Check sheet for the modelled part. Datum: model origin and axes. Units: mm. A direction names the side the tool comes from. Round coordinates to 2 decimals unless told otherwise and drop trailing zeros. Order: outer loops, then holes, each group sorted by start corner. A loop starts at its lowest first (then second) coordinate and runs counter-clockwise, first axis right, second up.
```python
from build123d import *

# Parameters (mm, degrees)
F0_W      = 50.8
F0_H      = 457.2
F1_DEPTH  = 25.4
F2_W      = 25.4
F2_H      = 50.8
F3_DEPTH  = 25.4
F4_W      = 25.4
F4_H      = 50.8
F5_DEPTH  = 431.8
F6_W      = 25.4
F6_H      = 50.8
F7_DEPTH  = 50.8
F8_W      = 50.8
F8_H      = 25.4
F9_DEPTH  = 406.4
F10_W     = 25.4
F10_H     = 50.8
F11_DEPTH = 25.4
F12_W     = 25.4
F12_H     = 50.8
F13_DEPTH = 431.8
F14_W     = 50.8
F14_H     = 50.8
F15_DEPTH = 25.4
F16_W     = 25.4
F16_H     = 50.8
F17_DEPTH = 381
F18_W     = 76.2
F18_H     = 50.8
F19_DEPTH = 25.4
F20_W     = 50.8
F20_H     = 25.4
F21_DEPTH = 406.4
F22_W     = 25.4
F22_H     = 50.8
F23_DEPTH = 406.4
F24_W     = 25.4
F24_H     = 50.8
F25_DEPTH = 431.8
F26_W     = 25.4
F26_H     = 50.8
F27_DEPTH = 406.4
F28_W     = 25.4
F28_H     = 50.8
F29_DEPTH = 25.4
F30_W     = 25.4
F30_H     = 50.8
F31_DEPTH = 431.8
F32_W     = 25.4
F32_H     = 50.8
F33_DEPTH = 431.8
F34_W     = 50.8
F34_H     = 50.8
F35_DEPTH = 25.4
F36_W     = 50.8
F36_H     = 25.4
F37_DEPTH = 406.4


with BuildPart() as f1:
    # F0 (on Front) → F1 (new body)
    with BuildSketch(Plane.XZ):
        with Locations((25.4, 228.6)):
            Rectangle(F0_W, F0_H)
    extrude(amount=F1_DEPTH)

    # F2 (on face) → F3 (join)
    with BuildSketch(Plane.YZ.offset(50.8)):
        with Locations((-12.7, 431.8)):
            Rectangle(F2_W, F2_H)
    extrude(amount=F3_DEPTH)

    # F4 (on face) → F5 (join)
    with BuildSketch(Plane.XZ.offset(25.4)):
        with Locations((63.5, 431.8)):
            Rectangle(F4_W, F4_H)
    extrude(amount=F5_DEPTH)

    # F6 (on face) → F7 (join)
    with BuildSketch(Plane(origin=(50.8, 0, 0), x_dir=(0, -1, 0), z_dir=(-1, 0, 0))):
        with Locations((444.5, 431.8)):
            Rectangle(F6_W, F6_H)
    extrude(amount=F7_DEPTH)

    # F8 (on face) → F9 (join)
    with BuildSketch(Plane(origin=(0, 0, 406.4), x_dir=(1, 0, 0), z_dir=(0, 0, -1))):
        with Locations((25.4, 444.5)):
            Rectangle(F8_W, F8_H)
    extrude(amount=F9_DEPTH)

    # F10 (on face) → F11 (join)
    with BuildSketch(Plane.YZ.offset(50.8)):
        with Locations((-12.7, 25.4)):
            Rectangle(F10_W, F10_H)
    extrude(amount=F11_DEPTH)

    # F12 (on face) → F13 (join)
    with BuildSketch(Plane.XZ.offset(25.4)):
        with Locations((63.5, 25.4)):
            Rectangle(F12_W, F12_H)
    extrude(amount=F13_DEPTH)

    # F14 (on face) → F15 (join)
    with BuildSketch(Plane(origin=(0, -431.8, 0), x_dir=(-1, 0, 0), z_dir=(0, 1, 0))):
        with Locations((-25.4, 431.8)):
            Rectangle(F14_W, F14_H)
    extrude(amount=F15_DEPTH)

    # F16 (on face) → F17 (join)
    with BuildSketch(Plane(origin=(0, 0, 0), x_dir=(0, -1, 0), z_dir=(-1, 0, 0))):
        with Locations((419.1, 431.8)):
            Rectangle(F16_W, F16_H)
    extrude(amount=F17_DEPTH)

    # F18 (on face) → F19 (join)
    with BuildSketch(Plane.XZ.offset(431.8)):
        with Locations((-342.9, 431.8)):
            Rectangle(F18_W, F18_H)
    extrude(amount=F19_DEPTH)

    # F20 (on face) → F21 (join)
    with BuildSketch(Plane(origin=(0, 0, 406.4), x_dir=(1, 0, 0), z_dir=(0, 0, -1))):
        with Locations((-330.2, 444.5)):
            Rectangle(F20_W, F20_H)
    extrude(amount=F21_DEPTH)

    # F22 (on face) → F23 (join)
    with BuildSketch(Plane(origin=(0, -406.4, 0), x_dir=(-1, 0, 0), z_dir=(0, 1, 0))):
        with Locations((368.3, 431.8)):
            Rectangle(F22_W, F22_H)
    extrude(amount=F23_DEPTH)

    # F24 (on face) → F25 (join)
    with BuildSketch(Plane(origin=(50.8, 0, 0), x_dir=(0, -1, 0), z_dir=(-1, 0, 0))):
        with Locations((419.1, 25.4)):
            Rectangle(F24_W, F24_H)
    extrude(amount=F25_DEPTH)

    # F26 (on face) → F27 (join)
    with BuildSketch(Plane(origin=(0, -406.4, 0), x_dir=(-1, 0, 0), z_dir=(0, 1, 0))):
        with Locations((368.3, 25.4)):
            Rectangle(F26_W, F26_H)
    extrude(amount=F27_DEPTH)

    # F28 (on face) → F29 (join)
    with BuildSketch(Plane(origin=(-355.6, 0, 0), x_dir=(0, -1, 0), z_dir=(-1, 0, 0))):
        with Locations((444.5, 25.4)):
            Rectangle(F28_W, F28_H)
    extrude(amount=F29_DEPTH)

    # F30 (on face) → F31 (join)
    with BuildSketch(Plane(origin=(50.8, 0, 0), x_dir=(0, -1, 0), z_dir=(-1, 0, 0))):
        with Locations((38.1, 25.4)):
            Rectangle(F30_W, F30_H)
    extrude(amount=F31_DEPTH)

    # F32 (on face) → F33 (join)
    with BuildSketch(Plane(origin=(50.8, 0, 0), x_dir=(0, -1, 0), z_dir=(-1, 0, 0))):
        with Locations((38.1, 431.8)):
            Rectangle(F32_W, F32_H)
    extrude(amount=F33_DEPTH)

    # F34 (on face) → F35 (join)
    with BuildSketch(Plane(origin=(0, -25.4, 0), x_dir=(-1, 0, 0), z_dir=(0, 1, 0))):
        with Locations((330.2, 25.4)):
            Rectangle(F34_W, F34_H)
    extrude(amount=F35_DEPTH)

    # F36 (on face) → F37 (join)
    with BuildSketch(Plane.XY.offset(50.8)):
        with Locations((-330.2, -12.7)):
            Rectangle(F36_W, F36_H)
    extrude(amount=F37_DEPTH)


solid = f1.part
```
Item 1: Sectioned sample at C-C (z = 360.5). Record the cut outline in (x, y).
Answer:
outline: (-355.6, -457.2) - (-304.8, -457.2) - (-304.8, -431.8) - (-355.6, -431.8) - close; (-355.6, -25.4) - (-304.8, -25.4) - (-304.8, 0) - (-355.6, 0) - close; (0, -457.2) - (50.8, -457.2) - (50.8, -431.8) - (0, -431.8) - close; (0, -25.4) - (50.8, -25.4) - (50.8, 0) - (0, 0) - close
Item 2: Sectioned sample at A-A (y = -303.5). Record the cut outline in (x, z), and give its area (3 significant figures).
Answer:
outline: (-381, 0) - (-355.6, 0) - (-355.6, 50.8) - (-381, 50.8) - close; (-381, 406.4) - (-355.6, 406.4) - (-355.6, 457.2) - (-381, 457.2) - close; (50.8, 0) - (76.2, 0) - (76.2, 50.8) - (50.8, 50.8) - close; (50.8, 406.4) - (76.2, 406.4) - (76.2, 457.2) - (50.8, 457.2) - close
area: 5,160 mm2
Item 3: Access from +Z, -Z, +X, -X, +Y, -Y to the whole of each face (thin tool, end or side, straight path). Record for faces 1 (the flat face through (-150, -406.4, 25)), 2 (the flat face through (-355.6, -13, 226)), 3 (the flat face through (-304.8, -13, 225)), 4 (the flat face through (50.8, -444, 231)), 5 (the flat face through (-331, -25.4, 226)).
Answer:
face 1: +Z, -Z
face 2: -X, +Y, -Y
face 3: +Z, -Z, +Y
face 4: +X, +Y, -Y
face 5: +X, -X
Item 4: Sectioned sample at B-B (x = -344). Record the cut outline in (y, z).
Answer:
outline: (-457.2, 0) - (-406.4, 0) - (-406.4, 50.8) - (-431.8, 50.8) - (-431.8, 406.4) - (-406.4, 406.4) - (-406.4, 457.2) - (-457.2, 457.2) - close; (-50.8, 0) - (0, 0) - (0, 457.2) - (-50.8, 457.2) - (-50.8, 406.4) - (-25.4, 406.4) - (-25.4, 50.8) - (-50.8, 50.8) - close
Item 5: Release check for a two-part mould opening along Y. For faces 6 (the flat face through (76.2, -225, 431)), 7 (the flat face through (-334, -457.2, 225)), 8 (the flat face through (50.8, -226, 25)) record: released by +Y, released by -Y, zero draft, split by the parting line, or undercut.
Answer:
face 6: zero draft
face 7: released by -Y
face 8: undercut
Item 6: Scan lines: line 1 along X through (y, z) = (-149.5, 414); line 2 along Y through (x, z) = (-325.5, 423); line 3 along Y through (x, z) = (-87, 25.5). Record each from-to range of solid material in increasing order.
Answer:
line 1: x = -381 to -355.6, 50.8 to 76.2
line 2: y = -457.2 to -406.4, -50.8 to 0
line 3: y = -431.8 to -406.4, -50.8 to -25.4
Item 7: Sectioned sample at D-D (y = -41). Record the cut outline in (x, z).
Answer:
outline: (-381, 0) - (76.2, 0) - (76.2, 50.8) - (-381, 50.8) - close; (-381, 406.4) - (76.2, 406.4) - (76.2, 457.2) - (-381, 457.2) - close
Item 8: Go/stop test with flat-tipped pins: P1, Ø20.5, axis at y = -14, z = 137, coming from the +X side; P2, Ø12.5, axis at y = -443, z = 315, coming from the -X side; P3, Ø15, axis at x = -83.5, z = 440, coming from the +Y side. Record where each tip stops, or that it passes through.
Answer:
P1: stops at x = 50.8
P2: stops at x = -355.6
P3: stops at y = -25.4
